Autodesk Fusion 360 part; units mm, degrees
sketch "Sketch1" plane through (0, 0, 0) normal (0, 0, 1) x (1, 0, 0)
  line L0 (0, 0) -> (140, 0)
  line L1 (140, 0) -> (140, 140)
  line L2 (140, 140) -> (0, 140)
  line L3 (0, 140) -> (0, 0)
  dimension "d1" = 140
  dimension "d2" = 140
extrude "Extrude1" add sketch "Sketch1" along normal blind 110
sketch "Sketch2" plane through (0, 0, 110) normal (0, 0, 1) x (-1, 0, 0)
  line L0 (0, -140) -> (0, 0)
  line L1 (0, 0) -> (-140, 0)
  line L2 (-140, 0) -> (-140, -140)
  line L3 (-140, -140) -> (0, -140)
  line L4 (0, -140) -> (-3, -140)
  line L5 (-3, -140) -> (-3, -137)
  line L6 (-3, -137) -> (0, -137)
  line L7 (0, -137) -> (0, -140)
  line L8 (-70, -140) -> (-70, 0)
  line L9 (0, -100) -> (-140, -100)
  line L10 (0, -60) -> (-140, -60)
  line L11 (-137, -137) -> (-140, -137)
  line L12 (-137, -140) -> (-137, -137)
  line L13 (-3, -63) -> (0, -63)
  line L14 (-3, -60) -> (-3, -63)
  line L15 (-137, -60) -> (-137, -63)
  line L16 (-137, -63) -> (-140, -63)
  line L17 (0, -100) -> (-3, -100)
  line L18 (-3, -100) -> (-3, -97)
  line L19 (-3, -97) -> (0, -97)
  line L20 (0, -97) -> (0, -100)
  line L21 (0, -100) -> (-140, -100)
  line L22 (-140, -100) -> (-140, -97)
  line L23 (-140, -97) -> (0, -97)
  line L24 (0, -97) -> (0, -100)
  line L25 (-140, -60) -> (0, -60)
  line L26 (0, -60) -> (0, -63)
  line L27 (0, -63) -> (-140, -63)
  line L28 (-140, -63) -> (-140, -60)
  line L29 (-140, -140) -> (0, -140)
  line L30 (0, -140) -> (0, -137)
  line L31 (0, -137) -> (-140, -137)
  line L32 (-140, -137) -> (-140, -140)
  line L33 (0, -140) -> (-3, -140)
  line L34 (-3, -140) -> (-3, 0)
  line L35 (-3, 0) -> (0, 0)
  line L36 (0, 0) -> (0, -140)
  line L37 (-140, -140) -> (-137, -140)
  line L38 (-137, -140) -> (-137, 0)
  line L39 (-137, 0) -> (-140, 0)
  line L40 (-140, 0) -> (-140, -140)
  dimension "d5" = 3
  dimension "d6" = 3
  dimension "d7" = 3
  dimension "d8" = 3
extrude "Extrude2" cut sketch "Sketch2" against normal blind 110 contours L8 L9 L21 L31 L34 | L8 L9 L21 L31 L38 | L8 L23 L27 L34 | L8 L23 L27 L38 | L1 L8 L10 L25 L34 | L1 L8 L10 L25 L38
sketch "Sketch3" plane through (140, 0, 0) normal (1, 0, 0) x (0, 1, 0)
  line L0 (0, 0) -> (140, 0)
  line L1 (140, 0) -> (140, 110)
  line L2 (140, 110) -> (0, 110)
  line L3 (0, 110) -> (0, 0)
  line L4 (0, 110) -> (10, 110)
  line L5 (10, 110) -> (10, 100)
  line L6 (10, 100) -> (0, 100)
  line L7 (0, 100) -> (0, 110)
  line L8 (0, 0) -> (10, 0)
  line L9 (10, 0) -> (10, 10)
  line L10 (10, 10) -> (0, 10)
  line L11 (0, 10) -> (0, 0)
  line L12 (60, 110) -> (50, 110)
  line L13 (50, 110) -> (50, 100)
  line L14 (50, 100) -> (60, 100)
  line L15 (60, 100) -> (60, 110)
  line L16 (60, 0) -> (50, 0)
  line L17 (50, 0) -> (50, 10)
  line L18 (50, 10) -> (60, 10)
  line L19 (60, 10) -> (60, 0)
  line L20 (50, 10) -> (10, 10)
  line L21 (10, 10) -> (10, 100)
  line L22 (10, 100) -> (50, 100)
  line L23 (50, 100) -> (50, 10)
  line L24 (60, 100) -> (60, 10)
extrude "Extrude3" cut sketch "Sketch3" against normal blind 140 contours L3 L6 L10 L21 | L20 L21 L22 L23 | L14 L18 L23 L24
sketch "Sketch5" plane through (0, 0, 0) normal (-1, 0, 0) x (0, -1, 0)
  line L0 (0, 10) -> (-60, 10)
  line L1 (-60, 10) -> (-60, 100)
  line L2 (-60, 100) -> (0, 100)
  line L3 (0, 100) -> (0, 110)
  line L4 (0, 110) -> (-140, 110)
  line L5 (-140, 110) -> (-140, 0)
  line L6 (-140, 0) -> (0, 0)
  line L7 (0, 0) -> (0, 10)
  line L8 (-136.5713, 0) -> (-100, 0)
  line L9 (-100, 0) -> (-100, 110)
  line L10 (-100, 110) -> (-136.5713, 110)
  line L11 (-136.5713, 110) -> (-136.5713, 0)
  line L12 (-136.5713, 5.3179) -> (-100, 5.3179)
  line L13 (-100, 5.3179) -> (-100, 105)
  line L14 (-100, 105) -> (-136.5713, 105)
  line L15 (-136.5713, 105) -> (-136.5713, 5.3179)
  line L16 (-96.7286, 0) -> (-63.0271, 0)
  line L17 (-63.0271, 0) -> (-63.0271, 110)
  line L18 (-63.0271, 110) -> (-96.7286, 110)
  line L19 (-96.7286, 110) -> (-96.7286, 0)
  line L20 (-96.7286, 5.3179) -> (-63.0271, 5.3179)
  line L21 (-63.0271, 5.3179) -> (-63.0271, 104.8767)
  line L22 (-63.0271, 104.8767) -> (-96.7286, 104.8767)
  line L23 (-96.7286, 104.8767) -> (-96.7286, 5.3179)
extrude "Extrude4" cut sketch "Sketch5" against normal blind 140 contours L17 L19 L20 L21 L22 L23 | L9 L11 L12 L13 L14 L15
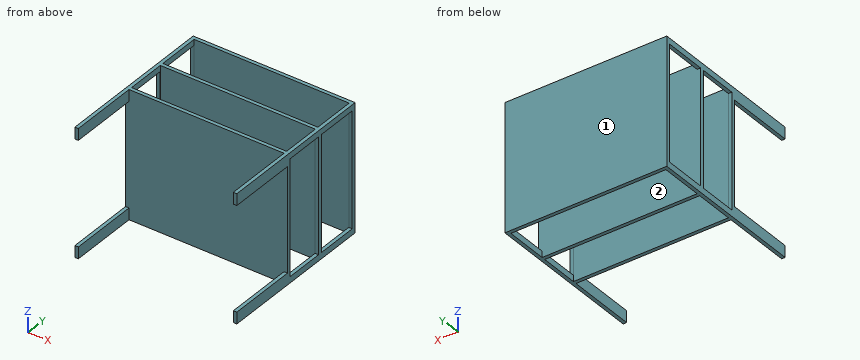
Verification items for the finished model (mm, model axes). Face numbers are marked on the shaded views. Give positions to 0.01 mm unless a question says otherwise; leave off trailing zeros. Loops run counter-clockwise (first coordinate to the right, second up) from the corner with the lowest first, then second, coordinate; pieces in that order, holes last.
1) Thickness scan on line 1 along Y through (x, z) = (78, 89). Record the ranges inside material, lowest first.
2) Draft check along Y on the marked faces 1 and 2. Enter one of: pulls with the +Y half, pulls with the -Y half, needs draft (parallel to the pull), parting line crosses it, or undercut.
3) Sectioned sample at C-C, the plane x = 27. Enter the section's corners in (y, z), then the cut area to 3 significant figures.
4) Sectioned sample at D-D, the plane y = 35.5. Enter the section's corners in (x, z), then the cut area to 3 significant figures.
5) Sectioned sample at A-A, the plane z = 59. Count the separate pieces of the cut face and the enclosed holes in it, then the cut area to 3 significant figures.
6) Sectioned sample at B-B, the plane y = 88. Enter the section's corners in (x, z), then the cut area to 3 significant figures.
7) Depth check by flat-ended pin: pin 1 Ø3.5 at (x, z) = (2, 52.5) entering from -Y. Enter the tip coordinate at first touch or a pass-through.
Answers:
1. line 1: y = 60 to 63, 97 to 100, 137 to 140
2. face 1: pulls with the +Y half
2. face 2: undercut
3. outline: (60, 0) - (63, 0) - (63, 110) - (60, 110) - close; (97, 0) - (100, 0) - (100, 110) - (97, 110) - close; (137, 0) - (140, 0) - (140, 110) - (137, 110) - close
3. area: 990 mm2
4. outline: (0, 0) - (3, 0) - (3, 10) - (0, 10) - close; (0, 100) - (3, 100) - (3, 110) - (0, 110) - close; (137, 0) - (140, 0) - (140, 10) - (137, 10) - close; (137, 100) - (140, 100) - (140, 110) - (137, 110) - close
4. area: 120 mm2
5. separate pieces: 3
5. enclosed holes: 0
5. area: 1,260 mm2
6. outline: (0, 0) - (3, 0) - (3, 5.32) - (0, 5.32) - close; (0, 104.88) - (3, 104.88) - (3, 110) - (0, 110) - close; (137, 0) - (140, 0) - (140, 5.32) - (137, 5.32) - close; (137, 104.88) - (140, 104.88) - (140, 110) - (137, 110) - close
6. area: 62.6 mm2
7. pin 1: stops at y = 60
